For this review, use the dimensioned drawing (mm, ordinates from the lowest corner) and the shaded views. Round coordinates to 2 decimals unless told otherwise and drop trailing zeros. Order: outer loops, then holes, each group sorted by start corner. A loop starts at its lowest first (then second) coordinate and runs counter-clockwise, first axis right, second up. Notation, with made-up numbers: M 11.25,46 L 26.25,46 A24 cw 26.25,66 Z; hole C 14,-18.5 d6. An arc over 180 degrees is marked long. Answer as CSV lines item,"result". Start each with the question number.
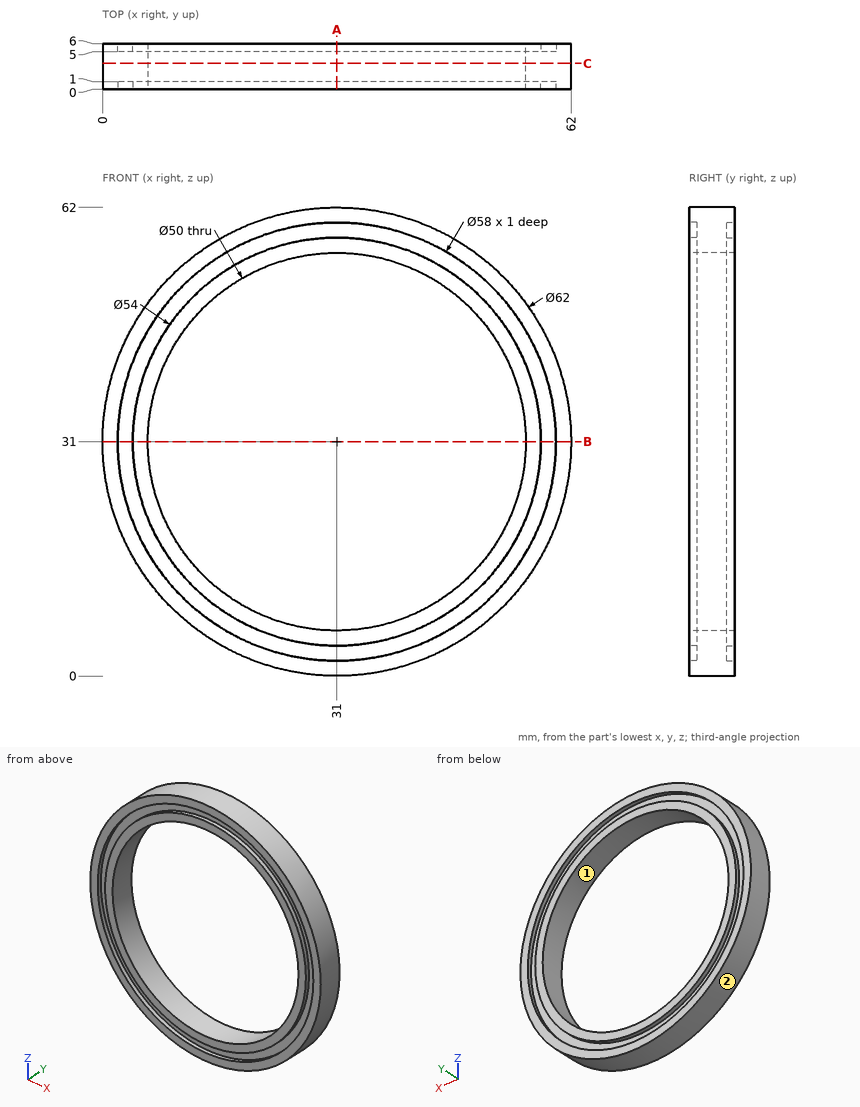
Item 1: Consider section C-C (y = 3.45). State the section outline as (x, z) points.
Item 2: Consider section B-B (z = 31). State the section outline as (x, y) points, and give its area (3 significant figures).
Item 3: For pin 1 (2 mm diameter, centred on y = 1.5, z = 16.5, fed in from -X); pin 2 (3 mm diameter, centred on x = 12, y = 4.5, fed in from -Z); pin 3 (2 mm diameter, centred on x = 31.5, y = 3, fed in from -Z); pin 4 (2 mm diameter, centred on x = 13.5, z = 17.5, fed in from +Y) (1 decimal), all flat-tipped, find the tip position at first contact; note any pin that passes through.
Item 4: Wall thickness on probe 1 along Z at (x, y) = (31, 5.25); probe 2 along X at (y, z) = (1.9, 31): over which ranges is each line inside the solid? List them lowest first. Write a range as [from, to].
Item 5: The part is to be moulded in two halves that separate along Z. For the marked faces 1 and 2, say which applies: +Z half, -Z half, draft (parallel to the pull), parting line (faces both ways), or undercut.
Item 6: Consider section A-A (x = 31). State the section outline as (y, z) points, and give its area (3 significant figures).
Reported:
1,outline,"C 31,31 d62; hole C 31,31 d50"
2,outline,"M 0,0 L 2,0 L 2,1 L 4,1 L 4,0 L 6,0 L 6,6 L 4,6 L 4,5 L 2,5 L 2,6 L 0,6 Z; M 56,0 L 58,0 L 58,1 L 60,1 L 60,0 L 62,0 L 62,6 L 60,6 L 60,5 L 58,5 L 58,6 L 56,6 Z"
2,area,"64.0 mm²"
3,pin 1,"stops at x = 3.09"
3,pin 2,"stops at z = 5.41"
3,pin 3,"stops at z = 0"
3,pin 4,"passes through"
4,probe 1,"z = [0, 2], [4, 6], [56, 58], [60, 62]"
4,probe 2,"x = [0, 6], [56, 62]"
5,face 1,"undercut"
5,face 2,"parting line"
6,outline,"M 0,0 L 6,0 L 6,2 L 5,2 L 5,4 L 6,4 L 6,6 L 0,6 L 0,4 L 1,4 L 1,2 L 0,2 Z; M 0,56 L 6,56 L 6,58 L 5,58 L 5,60 L 6,60 L 6,62 L 0,62 L 0,60 L 1,60 L 1,58 L 0,58 Z"
6,area,"64.0 mm²"
